from build123d import *

# Parameters (mm, degrees)
BOSS_EXTRUDE1_DEPTH = 10
BOSS_EXTRUDE1_DRAFT = -0.5
BOSS_EXTRUDE2_DEPTH = 10
SKETCH3_W           = 100
SKETCH3_H           = 2
SKETCH3_W_2         = 95
SKETCH3_W_3         = 90
SKETCH3_W_4         = 85
SKETCH3_W_5         = 80
CUT_EXTRUDE1_DEPTH  = 143.828568571
SKETCH4_R           = 70
CUT_EXTRUDE2_DEPTH  = 10
CUT_EXTRUDE2_DRAFT  = -2


with BuildPart() as part:
    # Sketch1 → Boss-Extrude1 (with draft: the straight prism first)
    with BuildSketch(Plane(origin=(0, 0, 0), x_dir=(1, 0, 0), z_dir=(0, 1, 0))):
        with BuildLine():
            ThreePointArc((-50, 74.833147735), (0, -90), (50, 74.833147735))
            Line((50, 74.833147735), (50, 70))
            Line((50, 70), (-50, 70))
            Line((-50, 70), (-50, 74.833147735))
        make_face()
    extrude(amount=-BOSS_EXTRUDE1_DEPTH)
    # Boss-Extrude1: the draft: its side faces are tilted about the plane it starts from
    boss_extrude1_sides = [part.faces().sort_by_distance(p)[0] for p in [
        (50, -5, -72.416573868),
        (0, -5, -70),
        (-50, -5, -72.416573868),
        (0, -5, 90),
    ]]
    draft(boss_extrude1_sides, Plane(origin=(0, 0, 0), x_dir=(1, 0, 0), z_dir=(0, 1, 0)), BOSS_EXTRUDE1_DRAFT)

    # Sketch2 → Boss-Extrude2 (add)
    with BuildSketch(Plane(origin=(0, 0, 0), x_dir=(1, 0, 0), z_dir=(0, 1, 0))):
        with BuildLine():
            Line((-40, 91.651513899), (-40, 80))
            Line((-40, 80), (40, 80))
            Line((40, 80), (40, 91.651513899))
            ThreePointArc((40, 91.651513899), (0, -100), (-40, 91.651513899))
        make_face()
    extrude(amount=BOSS_EXTRUDE2_DEPTH)

    # Sketch3 → Cut-Extrude1 (cut, through all)
    with BuildSketch(Plane(origin=(0, 10, 0), x_dir=(1, 0, 0), z_dir=(0, 1, 0))):
        with Locations((0, -19.17330362)):
            Rectangle(SKETCH3_W, SKETCH3_H)
        with Locations((0, -26.17330362)):
            Rectangle(SKETCH3_W_2, SKETCH3_H)
        with Locations((0, -33.17330362)):
            Rectangle(SKETCH3_W_3, SKETCH3_H)
        with Locations((0, -40.17330362)):
            Rectangle(SKETCH3_W_4, SKETCH3_H)
        with Locations((0, -47.17330362)):
            Rectangle(SKETCH3_W_5, SKETCH3_H)
    extrude(amount=-CUT_EXTRUDE1_DEPTH, mode=Mode.SUBTRACT)


with BuildPart() as cut_extrude2_tool:
    # Sketch4 → Cut-Extrude2 (with draft: the straight prism first)
    with BuildSketch(Plane(origin=(0, 10, 0), x_dir=(1, 0, 0), z_dir=(0, 1, 0))):
        Circle(SKETCH4_R)
    extrude(amount=-CUT_EXTRUDE2_DEPTH)
    # Cut-Extrude2: the draft: its side faces are tilted about the plane it starts from
    cut_extrude2_sides = [cut_extrude2_tool.faces().sort_by_distance(p)[0] for p in [
        (-70, 5, 0),
    ]]
    draft(cut_extrude2_sides, Plane(origin=(0, 10, 0), x_dir=(1, 0, 0), z_dir=(0, 1, 0)), CUT_EXTRUDE2_DRAFT)


with BuildPart() as part_1:
    add(part.part)

    # Cut-Extrude2: cut by cut_extrude2_tool
    add(cut_extrude2_tool.part, mode=Mode.SUBTRACT)


solid = part_1.part
The listing builds one solid part. Answer for the finished solid, in the listing's coordinates (mm). A direction names the side the tool comes from. Round coordinates to 2 decimals unless told otherwise and drop trailing zeros. Order: outer loops, then holes, each group sorted by start corner. A loop starts at its lowest first (then second) coordinate and runs counter-clockwise, first axis right, second up. Notation, with made-up numbers: M -35.75,88.25 L 23.25,88.25 A35 cw 23.25,121.25 Z; hole C 43.25,-26 d7. An arc over 180 degrees is marked long. Answer in a Markdown table with one row per item. Add a question column.
1) Determine the mould class of faces 4 (the face through (-1, -10, 6)), 5 (the face through (-3.21, -6.04, 89.89)), 6 (the face through (-1, -5, 34.173)) for opening direction X: pulls with the +X half, pulls with the -X half, needs draft (parallel to the pull), parting line crosses it, or undercut.
2) The part is cut by section B-B on x = 0. Count the separate pieces of the cut face and the enclosed holes in it, plus the area to 3 significant figures.
3) The part is cut by section A-A on y = -4. Determine the outline of the cut face in (x, z).
4) Consider line 1 along Z through (x, y) = (-3.5, -1.5); line 2 along Z through (x, y) = (-26, -9); line 3 along Y through (x, z) = (87, 48.5). Determine where each line is inside the solid, lowest interval first. Write a range as from..to.
5) Which of the six approach directions +Z, -Z, +X, -X, +Y, -Y give full straight-line access (tool end or side, diameter ignored) to faces 1 (the face through (-1, -5, 20.173)), 2 (the face through (-1, 0, -1)), 3 (the face through (40, 5, -86))?
6) Flat-ended cylindrical pins translate along their axes: pin 1 Ø10 at (y, z) = (-6.5, 6.5) entering from -X; pin 2 Ø3 at (y, z) = (7, -83.5) entering from +X; pin 3 Ø3 at (x, y) = (14.5, -6.5) entering from -Z. Find the tip coordinate at first contact, or state that the pin passes through.
Findings below:
| question | item | result |
|---|---|---|
| 1 | face 4 | needs draft |
| 1 | face 5 | parting line crosses it |
| 1 | face 6 | undercut |
| 2 | separate pieces | 6 |
| 2 | enclosed holes | 0 |
| 2 | area | 1,900 mm² |
| 3 | outline | M -50.03,-74.77 L -50.03,-69.97 L 50.03,-69.97 L 50.03,-74.77 A89.97 ccw long Z; hole M -50,18.17 L 50,18.17 L 50,20.17 L -50,20.17 Z; hole M -47.5,25.17 L 47.5,25.17 L 47.5,27.17 L -47.5,27.17 Z; hole M -45,32.17 L 45,32.17 L 45,34.17 L -45,34.17 Z; hole M -42.5,39.17 L 42.5,39.17 L 42.5,41.17 L -42.5,41.17 Z; hole M -40,46.17 L 40,46.17 L 40,48.17 L -40,48.17 Z |
| 4 | line 1 | z = -69.99..18.17, 20.17..25.17, 27.17..32.17, 34.17..39.17, 41.17..46.17, 48.17..89.92 |
| 4 | line 2 | z = -69.92..18.17, 20.17..25.17, 27.17..32.17, 34.17..39.17, 41.17..46.17, 48.17..86.08 |
| 4 | line 3 | y = 0..10 |
| 5 | face 1 | +Y, -Y |
| 5 | face 2 | +Y |
| 5 | face 3 | -Z, +Y, -Y |
| 6 | pin 1 | stops at x = -89.94 |
| 6 | pin 2 | stops at x = 57.24 |
| 6 | pin 3 | stops at z = -69.96 |
